Input: part model. Units: mm. Frame: model coordinates. A direction names the side the tool comes from. Round coordinates to 2 decimals unless told otherwise and drop trailing zeros. Order: outer loops, then holes, each group sorted by start corner. A loop starts at its lowest first (then second) coordinate and runs counter-clockwise, first axis right, second up. Notation, with made-up numbers: M 6,57 L 46,57 A5 cw 46,65 Z; hole C -38,5.5 d11. An arc over 180 degrees is marked long. One line per question, with ' | ' between items.
```python
from build123d import *

# Parameters (mm, degrees)
SKETCH001_W  = 8.5
SKETCH001_H  = 1.51
POCKET_DEPTH = 1.3


with BuildPart() as part:
    # Sketch → Revolution (revolve)
    with BuildSketch(Plane.YZ):
        with BuildLine():
            Line((0, 3.503122), (0, 0))
            Line((0, 0), (23.3, 0))
            Line((23.3, 0), (23.3, 2.01))
            Line((23.3, 2.01), (23.017098, 2.5))
            Line((23.017098, 2.5), (3.3, 2.5))
            Line((3.3, 2.5), (3.3, 4.25))
            Line((3.3, 4.25), (0.456422, 4.001219))
            ThreePointArc((0.456422, 4.001219), (0.131361, 3.840917), (0, 3.503122))
        make_face()
    revolve(axis=Axis((0, 0, 0), (0, 1, 0)))

    # Sketch001 → Pocket (cut)
    with BuildSketch(Plane(origin=(0, 0, 0), x_dir=(0, 0, -1), z_dir=(0, -1, 0))):
        Rectangle(SKETCH001_W, SKETCH001_H)
    extrude(amount=-POCKET_DEPTH, mode=Mode.SUBTRACT)


solid = part.part
```
Item 1: Line query: line 1 along Y through (x, z) = (3, -1.5); line 2 along Y through (x, z) = (2, -0.25); line 3 along Z through (x, y) = (2, 9). Output: solid intervals per line, ascending. Write a range as from..to.
Report:
line 1: 0..3.3 | line 2: 0..23.3 | line 3: -1.5..1.5
Item 2: Access query for faces 1 (the flat face through (0, 23.3, 0)), 2 (the flat face through (-2, 3.3, -2)), 3 (the flat face through (-0.755, 1, 0)). Directions: +Z, -Z, +X, -X, +Y, -Y. A direction counts if a zero-diameter tool reaches every point of the face in a straight line with its end or side. Return the directions, or none.
Report:
face 1: +Z, -Z, +X, -X, +Y | face 2: +Y | face 3: +Z, -Z, -Y
Item 3: First-contact query: pin 1 (1.5 mm diameter, centred on y = 17, z = 1, fed in from -X); pin 2 (1 mm diameter, centred on x = 2.5, y = 21, fed in from +Z); pin 3 (1.2 mm diameter, centred on x = 0, z = 0.5, fed in from -Y). Flat tips, straight axial feed; report the tip coordinate or a pass-through.
Report:
pin 1: x = -2.49 | pin 2: z = 1.5 | pin 3: y = 1.3
Item 4: Section query C-C, the plane y = 20.5. Return loops of the section in (x, z), plus the area to 3 significant figures.
Report:
outline: C 0,0 d5 | area: 19.6 mm²
Item 5: Section query A-A, the plane z = 0. Return loops of the section in (x, y) (3 decimals).
Report:
outline: M -4.25,3.3 L -4.001,0.456 A0.5 ccw -3.503,0 L -0.755,0 L -0.755,1.3 L 0.755,1.3 L 0.755,0 L 3.503,0 A0.5 ccw 4.001,0.456 L 4.25,3.3 L 2.5,3.3 L 2.5,23.017 L 2.01,23.3 L -2.01,23.3 L -2.5,23.017 L -2.5,3.3 Z
Item 6: Section query B-B, the plane x = 0. Return loops of the section in (y, z), plus the area to 3 significant figures.
Report:
outline: M 1.3,-4.08 L 3.3,-4.25 L 3.3,-2.5 L 23.02,-2.5 L 23.3,-2.01 L 23.3,2.01 L 23.02,2.5 L 3.3,2.5 L 3.3,4.25 L 1.3,4.08 Z | area: 117 mm²
Item 7: Mould query, pull axis X, two halves, no side actions, for faces 4 (the flat face through (0, 1.3, 0)), 5 (the cylindrical face through (-2.44, 13.02, -0.54)), 6 (the flat face through (2, 0, 0)). Classes: +X half, -X half, draft (parallel to the pull), parting line (faces both ways), or undercut.
Report:
face 4: undercut | face 5: parting line | face 6: draft
